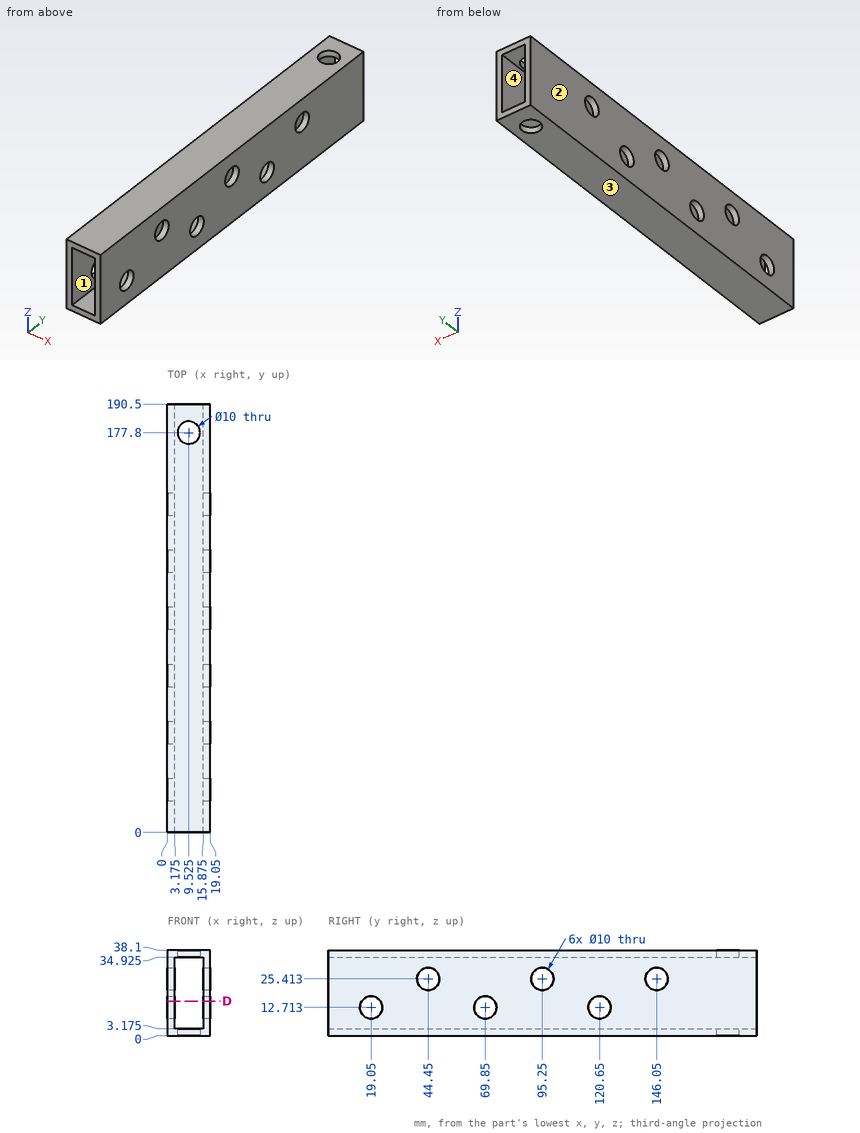
Geometry: see drawing. Coordinates: mm, zero at the bounding-box minimum. Round coordinates to 2 decimals unless told otherwise and drop trailing zeros. One line per question, with ' | ' between items. Start each with the question number.
1. Line query: line 1 along Z through (x, y) = (17.8, 19.05); line 2 along Z through (x, y) = (17.3, 44.45). Output: solid intervals per line, ascending. Write a range as [from, to].
2. Section D-D on z = 15.5. Count the separate pieces of the cut face and the enclosed holes in it, and give its area (3 significant figures).
3. Mould query, pull axis Z, two halves, no side actions, for the marked faces 1, 2, 3 and 4. Classes: pulls with the +Z half, pulls with the -Z half, needs draft (parallel to the pull), parting line crosses it, or undercut.
Returned:
1) line 1: z = [0, 7.71], [17.71, 38.1] | line 2: z = [0, 20.41], [30.41, 38.1]
2) separate pieces: 8 | enclosed holes: 0 | area: 1,050 mm2
3) face 1: undercut | face 2: needs draft | face 3: pulls with the -Z half | face 4: undercut
